Read the model definition and answer for the solid it produces. Units are mm, in the model's axes. A direction names the side the tool comes from. Round coordinates to 2 decimals unless told otherwise and drop trailing zeros. Order: outer loops, then holes, each group sorted by start corner. A loop starts at its lowest first (then second) coordinate and runs counter-clockwise, first axis right, second up.
from build123d import *

# Parameters (mm, degrees)
BOSS_EXTRUDE1_DEPTH = 1.524


with BuildPart() as part:
    # Sketch1 → Boss-Extrude1 (new body)
    with BuildSketch(Plane(origin=(0, 0, 0), x_dir=(0, 0, -1), z_dir=(1, 0, 0))):
        with BuildLine():
            Line((13.407652518, 17.110478898), (3.184449025, 10.435661085))
            Line((3.184449025, 10.435661085), (4.017618802, 9.159571698))
            Line((4.017618802, 9.159571698), (14.415583003, 15.948492286))
            ThreePointArc((14.415583003, 15.948492286), (21.092922372, 6.750259445), (26.29476658, -3.355934957))
            ThreePointArc((26.29476658, -3.355934957), (29.972883945, -9.528005236), (34.723111664, -14.918583638))
            ThreePointArc((34.723111664, -14.918583638), (36.135111524, -15.61884561), (37.536333073, -16.340433168))
            Line((37.536333073, -16.340433168), (17.883159134, -31.731702551))
            Line((17.883159134, -31.731702551), (18.82281135, -32.931548254))
            Line((18.82281135, -32.931548254), (39.005018059, -17.125969921))
            ThreePointArc((39.005018059, -17.125969921), (43.071954568, -19.463822973), (47.029287435, -21.982760456))
            ThreePointArc((47.029287435, -21.982760456), (47.121340823, -22.294468188), (46.831491474, -22.44151543))
            ThreePointArc((46.831491474, -22.44151543), (40.524268055, -36.485757729), (51.747180655, -25.946875351))
            ThreePointArc((51.747180655, -25.946875351), (51.79176687, -25.624931868), (52.116458195, -25.610403262))
            ThreePointArc((52.116458195, -25.610403262), (55.970170844, -28.311608841), (59.322656596, -31.614403422))
            Line((59.322656596, -31.614403422), (38.521293058, -48.704406988))
            Line((38.521293058, -48.704406988), (39.48874306, -49.8819538))
            Line((39.48874306, -49.8819538), (60.451087926, -32.659691044))
            ThreePointArc((60.451087926, -32.659691044), (65.449164438, -37.690671834), (70.092626303, -43.050690343))
            ThreePointArc((70.092626303, -43.050690343), (72.914169877, -46.704495979), (75.570723168, -50.479959972))
            Line((75.570723168, -50.479959972), (60.910405453, -63.506128463))
            Line((60.910405453, -63.506128463), (61.922669103, -64.64538186))
            Line((61.922669103, -64.64538186), (76.419081079, -51.764848943))
            ThreePointArc((76.419081079, -51.764848943), (85.346593392, -68.759689082), (90.997112415, -87.10626103))
            ThreePointArc((90.997112415, -87.10626103), (91.213266354, -93.748148771), (89.779086784, -100.23694868))
            Line((89.779086784, -100.23694868), (86.156676546, -97.139104436))
            Line((86.156676546, -97.139104436), (85.16617589, -98.297329135))
            Line((85.16617589, -98.297329135), (72.942235832, -87.843553926))
            Line((72.942235832, -87.843553926), (71.951735177, -89.001778624))
            Line((71.951735177, -89.001778624), (88.527211746, -103.176938614))
            ThreePointArc((88.527211746, -103.176938614), (88.240593298, -103.735184094), (87.940907668, -104.286524891))
            ThreePointArc((87.940907668, -104.286524891), (81.546731579, -108.065445103), (75.104666757, -104.368753791))
            ThreePointArc((75.104666757, -104.368753791), (65.647792617, -97.564665833), (55.732787106, -91.447415868))
            Line((55.732787106, -91.447415868), (70.587569953, -96.632218566))
            Line((70.587569953, -96.632218566), (71.089783687, -95.193344922))
            Line((71.089783687, -95.193344922), (46.757147713, -86.700463003))
            ThreePointArc((46.757147713, -86.700463003), (46.008174549, -86.335839826), (45.257363435, -85.975016415))
            ThreePointArc((45.257363435, -85.975016415), (42.216480057, -84.561010059), (39.14738639, -83.209326015))
            ThreePointArc((39.14738639, -83.209326015), (27.255727661, -77.897933177), (18.352985242, -68.39195513))
            ThreePointArc((18.352985242, -68.39195513), (9.477657224, -55.283796186), (-4.522491883, -47.89521694))
            ThreePointArc((-4.522491883, -47.89521694), (-9.486665924, -44.951872039), (-13.595983785, -40.899735587))
            ThreePointArc((-13.595983785, -40.899735587), (-16.824505318, -30.34398814), (-13.595983785, -19.788240693))
            ThreePointArc((-13.595983785, -19.788240693), (-11.273947375, -10.645865952), (-13.295774557, -1.432447268))
            ThreePointArc((-13.295774557, -1.432447268), (-9.527302248, 1.055622975), (-6.46891992, 4.377997821))
            ThreePointArc((-6.46891992, 4.377997821), (-21.126971598, 6.251882407), (-31.581931465, -4.191476087))
            ThreePointArc((-31.581931465, -4.191476087), (-31.126828301, 3.888628011), (-26.369564479, 10.435661085))
            ThreePointArc((-26.369564479, 10.435661085), (-23.587438274, 13.654628259), (-21.440611016, 17.327924955))
            ThreePointArc((-21.440611016, 17.327924955), (-18.964873682, 20.882521181), (-15.438488132, 23.398278447))
            ThreePointArc((-15.438488132, 23.398278447), (-2.701283032, 25.730330795), (9.447763641, 21.249758643))
            ThreePointArc((9.447763641, 21.249758643), (11.467468523, 19.218156049), (13.407652518, 17.110478898))
        make_face()
    extrude(amount=BOSS_EXTRUDE1_DEPTH)


solid = part.part
Q1. Straight lines are drawn through the part: probe 1 along Y at (x, z) = (0.85, -67); probe 2 along Y at (x, z) = (0.15, 13); probe 3 along Y at (x, z) = (1.15, 14). For each, find the intervals that lie inside material, in ascending order.
Outcome:
probe 1: y = -98.48 to -95.38, -93.77 to -60.13, -58.1 to -39.4
probe 2: y = -41.62 to -18.55, -2.08 to -1.28, 6.93 to 24.41
probe 3: y = -40.27 to -20.41, 7.06 to 24.03
Q2. A cutting plane is placed at B-B, the plane y = -62. Give the vertices of the cut face in (x, z), plus the area to 3 significant figures.
Outcome:
outline: (0, -82.27) - (1.52, -82.27) - (1.52, -64.9) - (0, -64.9) - close; (0, -62.61) - (1.52, -62.61) - (1.52, -15.19) - (0, -15.19) - close
area: 98.7 mm2
Q3. For a pull along Z with two mould halves and no side action, classify faces 3 (the face through (0.8, 6.9, -21)), 4 (the face through (0.751, -95.99, -80.123)), 5 (the face through (0.751, 3.78, 31.165)), 6 (the face through (0.75, 6.32, 20.92)) as released by +Z, released by -Z, zero draft, split by the parting line, or undercut.
Outcome:
face 3: released by -Z
face 4: undercut
face 5: released by +Z
face 6: undercut
Q4. A cutting plane is placed at A-A, the plane z = -80. Give the vertices of the cut face in (x, y).
Outcome:
outline: (0, -107.91) - (1.52, -107.91) - (1.52, -95.88) - (0, -95.88) - close; (0, -93.88) - (1.52, -93.88) - (1.52, -57.7) - (0, -57.7) - close
Q5. A cutting plane is placed at C-C, the plane y = -28.5. Give the vertices of the cut face in (x, z).
Outcome:
outline: (0, -56.19) - (1.52, -56.19) - (1.52, -52.77) - (0, -52.77) - close; (0, -37.4) - (1.52, -37.4) - (1.52, -24.48) - (0, -24.48) - close; (0, -22.01) - (1.52, -22.01) - (1.52, 16.73) - (0, 16.73) - close
Q6. For faces 1 (the face through (0.751, -98.71, -87.993)), 2 (the face through (0.751, -45.001, 9.422)), determine the directions among +Z, -Z, +X, -X, +Y, -Y from which every point of the face is accessible in a straight line to the end or side of a thin tool.
Outcome:
face 1: +X, -X
face 2: +Z, +X, -X, -Y
